Design review of the part built by this model. Coordinates are the model's own, in mm. A direction names the side the tool comes from. Coordinates: 2 decimals unless noted, no trailing zeros. Write each loop counter-clockwise with the first axis right and the second up, starting at its lowest first coordinate (ties: lowest second). Pieces come first, ordered by that corner, then holes. Notation, with made-up numbers: (40.5, -38) - (91.5, -38) arc R20 ccw to (91.5, -20) - close; hole circle Ø9 at (22, 13). An arc over 180 degrees is marked (long way). One line per item, written item: value.
from build123d import *


with BuildPart() as part:
    # Sketch1 → Revolve1 (revolve)
    with BuildSketch(Plane.XY, mode=Mode.PRIVATE) as revolve1_sk:
        with BuildLine():
            Line((-9.740947322, 26.185345129), (-9.740947322, -26.185345129))
            Line((-9.740947322, -26.185345129), (-19.522320179, -26.185345129))
            Line((-19.522320179, -26.185345129), (-19.522320179, -16.409199987))
            ThreePointArc((-19.522320179, -16.409199987), (-23.579011192, -6.615481526), (-33.372729652, -2.558790514))
            Line((-33.372729652, -2.558790514), (-55.000709219, -2.558790514))
            ThreePointArc((-55.000709219, -2.558790514), (-64.79442768, -6.615481526), (-68.851118692, -16.409199987))
            Line((-68.851118692, -16.409199987), (-68.851118692, -26.185345129))
            Line((-68.851118692, -26.185345129), (-77.3516349, -26.185345129))
            Line((-77.3516349, -26.185345129), (-77.3516349, -17.373618967))
            Line((-77.3516349, -17.373618967), (-77.3516349, -17.233064019))
            Line((-77.3516349, -17.233064019), (-79.265002978, -17.233064019))
            Line((-79.265002978, -17.233064019), (-79.265002978, 17.233064019))
            Line((-79.265002978, 17.233064019), (-77.3516349, 17.233064019))
            Line((-77.3516349, 17.233064019), (-77.3516349, 17.373618967))
            Line((-77.3516349, 17.373618967), (-77.3516349, 26.185345129))
            Line((-77.3516349, 26.185345129), (-68.851118692, 26.185345129))
            Line((-68.851118692, 26.185345129), (-68.851118692, 16.409199987))
            ThreePointArc((-68.851118692, 16.409199987), (-64.79442768, 6.615481526), (-55.000709219, 2.558790514))
            Line((-55.000709219, 2.558790514), (-33.372729652, 2.558790514))
            ThreePointArc((-33.372729652, 2.558790514), (-23.579011192, 6.615481526), (-19.522320179, 16.409199987))
            Line((-19.522320179, 16.409199987), (-19.522320179, 26.185345129))
            Line((-19.522320179, 26.185345129), (-9.740947322, 26.185345129))
        make_face()
    revolve(revolve1_sk.sketch.rotate(Axis((0, 0, 0), (0, 1, 0)), 270), axis=Axis((0, 0, 0), (0, 1, 0)))


solid = part.part
1. Consider section B-B, the plane y = 12.5. Write out the cut boundary in (x, z) (3 decimals), then the cut area to 3 significant figures.
Answer block:
outline: circle Ø158.53 at (0, 0); circle Ø40.171 at (0, 0); hole circle Ø136.576 at (0, 0); hole circle Ø19.482 at (0, 0)
area: 6,060 mm^2
2. Mouldability with a two-part tool opening along Z and no side actions: class faces 1 (the face through (-20.68, -21.37, -65.67)), 2 (the face through (-65.223, -21.647, -41.584)), 3 (the face through (-5, 26.185, 9)) as released by +Z, released by -Z, zero draft, split by the parting line, or undercut.
Answer block:
face 1: undercut
face 2: split by the parting line
face 3: zero draft
3. Wall thickness on line 1 along X through (y, z) = (18, 0); line 2 along Z through (x, y) = (-11, -7.5); line 3 along X through (y, z) = (2.5, 0) (3 decimals): over which ranges is each line inside the solid? List them lowest first.
Answer block:
line 1: x = -77.35 to -68.85, -19.52 to -9.74, 9.74 to 19.52, 68.85 to 77.35
line 2: z = -78.5 to -64.68, -19.93 to 19.93, 64.68 to 78.5
line 3: x = -79.265 to -9.741, 9.741 to 79.265
4. Insertion check: pin 1 Ø5 at (x, y) = (-46, 10.5) entering from +Z; pin 2 Ø4 at (x, z) = (36, -3.5) entering from +Y; pin 3 Ø8 at (x, z) = (11.5, 32) entering from -Y. Each pin has a flat end and moves straight along its axis. Give the tip position at first contact, or say it passes through.
Answer block:
pin 1: stops at z = 66.26
pin 2: stops at y = 2.56
pin 3: stops at y = -2.97
5. Consider section A-A, the plane y = -21. Write out the cut boundary in (x, z).
Answer block:
outline: circle Ø154.7 at (0, 0); circle Ø39.04 at (0, 0); hole circle Ø137.7 at (0, 0); hole circle Ø19.48 at (0, 0)
6. For faces 4 (the face through (45.5, 26.185, 51.9)), 5 (the face through (-20.68, 21.23, -65.67)), 6 (the face through (24, -2.559, 24)), list the 3-axis set-ups (+Z, -Z, +X, -X, +Y, -Y) from which the entire face can be reached by the end or side of a thin tool; tool diameter is ignored.
Answer block:
face 4: +Z, -Z, +X, -X, +Y
face 5: +Y
face 6: -Y
